Read the model definition and answer for the solid it produces. Units are mm, in the model's axes. A direction names the side the tool comes from. Give positions to 0.01 mm unless a question says otherwise; leave off trailing zeros. Loops run counter-clockwise (first coordinate to the right, second up) from the corner with the lowest first, then second, coordinate; pieces in that order, holes last. Notation, with made-up numbers: (89.25, -16) -> (147.25, -16) arc R22 ccw to (147.25, -5) -> close; hole circle Ø3 at (37, 75.25). An arc over 180 degrees is marked (long way). One line per item, written item: value. Start each with the question number.
from build123d import *

# Parameters (mm, degrees)
F0_W     = 56
F0_H     = 35
F0_W_2   = 44.448143
F0_H_2   = 2
F1_DEPTH = 3
F2_DEPTH = 10
F3_R     = 1.5
F4_R     = 1
F5_R     = 3


with BuildPart() as f1:
    # F0 (on Top) → F1 (new body)
    with BuildSketch(Plane.XY):
        with Locations((-37.713654, 34.063472)):
            Rectangle(F0_W, F0_H)
        with Locations((-37.713654, 31.653472)):
            Rectangle(F0_W_2, F0_H_2, mode=Mode.SUBTRACT)
        with Locations((-37.713654, 36.473472)):
            Rectangle(F0_W_2, F0_H_2, mode=Mode.SUBTRACT)
    extrude(amount=F1_DEPTH)

    # F0 (on Top) → F2 (join)
    with BuildSketch(Plane.XY):
        with Locations((-37.713654, 31.653472)):
            Rectangle(F0_W_2, F0_H_2)
        with Locations((-37.713654, 36.473472)):
            Rectangle(F0_W_2, F0_H_2)
    extrude(amount=F2_DEPTH)

    # F3
    f3_edges = [f1.edges().sort_by_distance(p)[0] for p in [
        (-59.937726, 35.473472, 6.5),
        (-59.937726, 32.653472, 6.5),
        (-15.489583, 35.473472, 6.5),
        (-15.489583, 32.653472, 6.5),
    ]]
    fillet(f3_edges, radius=F3_R)

    # F4
    f4_edges = [f1.edges().sort_by_distance(p)[0] for p in [
        (-37.713654, 35.473472, 10),
        (-37.713654, 32.653472, 10),
    ]]
    fillet(f4_edges, radius=F4_R)

    # F5
    f5_edges = [f1.edges().sort_by_distance(p)[0] for p in [
        (-9.713654, 51.563472, 1.5),
        (-65.713654, 16.563472, 1.5),
        (-65.713654, 51.563472, 1.5),
        (-9.713654, 16.563472, 1.5),
    ]]
    fillet(f5_edges, radius=F5_R)


solid = f1.part
Item 1: Flat-ended cylindrical pins translate along their axes: pin 1 (2 mm diameter, centred on x = -24.5, z = 7, fed in from +Y); pin 2 (3.5 mm diameter, centred on x = -36.5, z = 6.5, fed in from -Y); pin 3 (3 mm diameter, centred on y = 37, z = 7.5, fed in from -X). Find the tip coordinate at first contact, or state that the pin passes through.
Item 2: Section A-A, the plane z = 6.75 is taken. Determine the outline of the cut face in (x, y).
Item 3: Consider L1, parallel to Y at x = -46, z = 4.75; L2, parallel to Z at x = -61, y = 40.5; L3, parallel to X at y = 36, z = 9. Determine where each line is inside the solid, lowest interval first. Write a range as [from, to].
Item 4: Section C-C, the plane y = 24 is taken. Determine the outline of the cut face in (x, z), plus the area to 3 significant figures.
Item 5: Section B-B, the plane x = -48.5 is taken. Determine the outline of the cut face in (y, z).
Item 6: Determine the mould class of faces 1 (the flat face through (-65.714, 34, 1)), 2 (the flat face through (-38, 30.653, 6)), 3 (the cylindrical face through (-59.51, 32.2, 6.04)) for opening direction Y: pulls with the +Y half, pulls with the -Y half, needs draft (parallel to the pull), parting line crosses it, or undercut.
Item 7: For faces 4 (the flat face through (-38, 35.473, 6)), 5 (the cylindrical face through (-15.94, 35.9, 6.04)), 6 (the cylindrical face through (-59.487, 35.901, 6.042)), 7 (the flat face through (-38, 37.473, 6)), determine the directions among +Z, -Z, +X, -X, +Y, -Y from which every point of the face is accessible in a straight line to the end or side of a thin tool.
Computed values:
1. pin 1: y = 37.47
1. pin 2: y = 30.65
1. pin 3: x = -59.94
2. outline: (-59.94, 30.65) -> (-15.49, 30.65) -> (-15.49, 31.15) arc R1.5 ccw to (-16.99, 32.65) -> (-58.44, 32.65) arc R1.5 ccw to (-59.94, 31.15) -> close; (-59.94, 36.97) arc R1.5 ccw to (-58.44, 35.47) -> (-16.99, 35.47) arc R1.5 ccw to (-15.49, 36.97) -> (-15.49, 37.47) -> (-59.94, 37.47) -> close
3. L1: [30.65, 32.65], [35.47, 37.47]
3. L2: [0, 3]
3. L3: [-59.58, -15.85]
4. outline: (-65.71, 0) -> (-9.71, 0) -> (-9.71, 3) -> (-65.71, 3) -> close
4. area: 168 mm²
5. outline: (16.56, 0) -> (51.56, 0) -> (51.56, 3) -> (37.47, 3) -> (37.47, 10) -> (36.47, 10) arc R1 ccw to (35.47, 9) -> (35.47, 3) -> (32.65, 3) -> (32.65, 9) arc R1 ccw to (31.65, 10) -> (30.65, 10) -> (30.65, 3) -> (16.56, 3) -> close
6. face 1: needs draft
6. face 2: pulls with the -Y half
6. face 3: undercut
7. face 4: +Z, +X, -X
7. face 5: +Z, +X
7. face 6: +Z, -X
7. face 7: +Z, +X, -X, +Y
